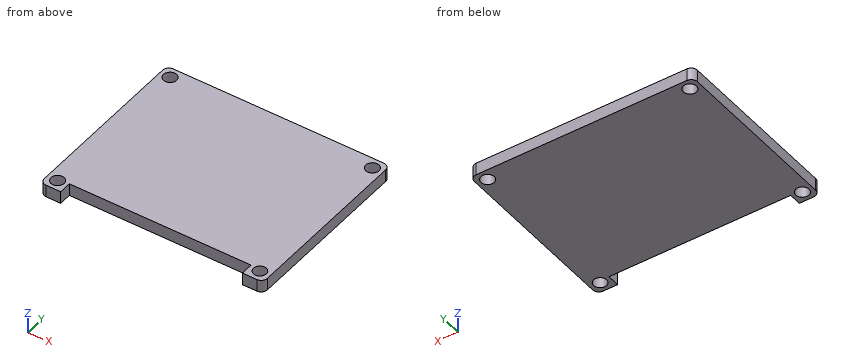
from build123d import *

# Parameters (mm, degrees)
SKETCH1_R           = 1.6
SKETCH1_R_2         = 1.559740896
BOSS_EXTRUDE1_DEPTH = 1.5


with BuildPart() as part:
    # Sketch1 → Boss-Extrude1 (new, symmetric)
    with BuildSketch(Plane.XY):
        with BuildLine():
            Line((22.828032498, -22.06376378), (21.828032498, -22.06376378))
            Line((21.828032498, -22.06376378), (21.828032498, -19.06376378))
            Line((21.828032498, -19.06376378), (-22.171967502, -19.06376378))
            Line((-22.171967502, -19.06376378), (-22.171967502, -22.06376378))
            Line((-22.171967502, -22.06376378), (-23.171967502, -22.06376378))
            Line((-23.171967502, -22.06376378), (-25.671967502, -22.06376378))
            ThreePointArc((-25.671967502, -22.06376378), (-26.732627674, -21.624423952), (-27.171967502, -20.56376378))
            Line((-27.171967502, -20.56376378), (-27.171967502, 20.43623622))
            ThreePointArc((-27.171967502, 20.43623622), (-26.732627674, 21.496896392), (-25.671967502, 21.93623622))
            Line((-25.671967502, 21.93623622), (25.328032498, 21.93623622))
            ThreePointArc((25.328032498, 21.93623622), (26.38869267, 21.496896392), (26.828032498, 20.43623622))
            Line((26.828032498, 20.43623622), (26.828032498, -20.56376378))
            ThreePointArc((26.828032498, -20.56376378), (26.38869267, -21.624423952), (25.328032498, -22.06376378))
            Line((25.328032498, -22.06376378), (22.828032498, -22.06376378))
        make_face()
        with Locations((-24.671967502, 19.43623622)):
            Circle(SKETCH1_R, mode=Mode.SUBTRACT)
        with Locations((24.328032498, 19.43623622)):
            Circle(SKETCH1_R, mode=Mode.SUBTRACT)
        with Locations((24.328032498, -19.56376378)):
            Circle(SKETCH1_R_2, mode=Mode.SUBTRACT)
        with Locations((-24.671967502, -19.56376378)):
            Circle(SKETCH1_R, mode=Mode.SUBTRACT)
    extrude(amount=BOSS_EXTRUDE1_DEPTH, both=True)


solid = part.part
Check sheet for the modelled part. Datum: model origin and axes. Units: mm. Coordinates: 2 decimals unless noted, no trailing zeros. Write each loop counter-clockwise with the first axis right and the second up, starting at its lowest first coordinate (ties: lowest second). Pieces come first, ordered by that corner, then holes.
Item 1: Cross-section at A-A on z = 1. Record the boundary of the cut face in (x, y).
Numbers:
outline: (-27.17, -20.56) arc R1.5 ccw to (-25.67, -22.06) - (-22.17, -22.06) - (-22.17, -19.06) - (21.83, -19.06) - (21.83, -22.06) - (25.33, -22.06) arc R1.5 ccw to (26.83, -20.56) - (26.83, 20.44) arc R1.5 ccw to (25.33, 21.94) - (-25.67, 21.94) arc R1.5 ccw to (-27.17, 20.44) - close; hole circle Ø3.2 at (-24.67, -19.56); hole circle Ø3.2 at (-24.67, 19.44); hole circle Ø3.2 at (24.33, 19.44); hole circle Ø3.12 at (24.33, -19.56)
Item 2: Scan lines: probe 1 along Y at (x, z) = (24.5, 0.4); probe 2 along X at (y, z) = (18.5, 0.5); probe 3 along Y at (x, z) = (24, 0.05). Record each from-to range of solid material in increasing order.
Numbers:
probe 1: y = -22.06 to -21.11, -18.01 to 17.85, 21.03 to 21.94
probe 2: x = -27.17 to -25.97, -23.37 to 23.03, 25.63 to 26.83
probe 3: y = -22.06 to -21.09, -18.04 to 17.87, 21 to 21.94
Item 3: Cross-section at B-B on x = 20. Record the boundary of the cut face in (y, z), then the cut area to 3 significant figures.
Numbers:
outline: (-19.06, -1.5) - (21.94, -1.5) - (21.94, 1.5) - (-19.06, 1.5) - close
area: 123 mm2
